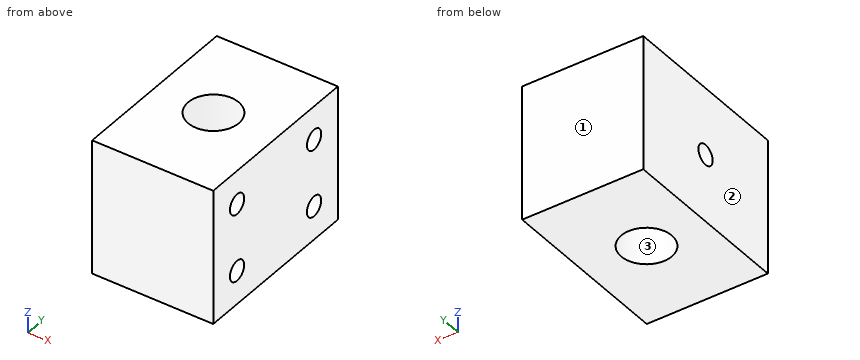
```python
from build123d import *

# Parameters (mm, degrees)
SKETCH1_W                            = 22.7965
SKETCH1_H                            = 33.263796714
SKETCH1_R                            = 4.7625
BOSS_EXTRUDE1_DEPTH                  = 25.4
SET_SCREW_10_24_TAPPED_HOLE1_REACH   = 49.658
SET_SCREW_10_24_TAPPED_HOLE1_BORE_R  = 1.89865
MOUNT_SCREW_10_24_TAPPED_HOLE2_D     = 3.7973
MOUNT_SCREW_10_24_TAPPED_HOLE2_DEPTH = 12.954
MOUNT_SCREW_10_24_TAPPED_HOLE2_TIP   = 1.140824014


with BuildPart() as part:
    # Sketch1 → Boss-Extrude1 (new body)
    with BuildSketch(Plane.XY):
        with Locations((11.39825, 16.631898357)):
            Rectangle(SKETCH1_W, SKETCH1_H)
        with Locations((11.1125, 16.631898357)):
            Circle(SKETCH1_R, mode=Mode.SUBTRACT)
    extrude(amount=BOSS_EXTRUDE1_DEPTH)

    # set screw #10-24 Tapped Hole1 bore → set screw #10-24 Tapped Hole1 (cut, up to next)
    with BuildSketch(Plane.ZY, mode=Mode.PRIVATE) as set_screw_10_24_tapped_hole1_sk1:
        with Locations((12.7, 16.631898357)):
            Circle(SET_SCREW_10_24_TAPPED_HOLE1_BORE_R)
    set_screw_10_24_tapped_hole1_tool1 = extrude(set_screw_10_24_tapped_hole1_sk1.sketch, amount=-SET_SCREW_10_24_TAPPED_HOLE1_REACH, mode=Mode.PRIVATE) & part.part
    add(set_screw_10_24_tapped_hole1_tool1.solids().sort_by_distance((0, 16.631898, 12.7))[0], mode=Mode.SUBTRACT)

    # mount screw #10-24 Tapped Hole2
    with Locations(Plane(origin=(22.7965, 0, 0), x_dir=(0, 0, -1), z_dir=(1, 0, 0))):
        with Locations((-19.05, 26.913796714), (-6.35, 26.913796714), (-19.05, 6.35), (-6.35, 6.35)):
            Hole(MOUNT_SCREW_10_24_TAPPED_HOLE2_D / 2, depth=MOUNT_SCREW_10_24_TAPPED_HOLE2_DEPTH)
            with Locations((0, 0, -(MOUNT_SCREW_10_24_TAPPED_HOLE2_DEPTH + MOUNT_SCREW_10_24_TAPPED_HOLE2_TIP / 2))):  # 118° drill point
                Cone(0, MOUNT_SCREW_10_24_TAPPED_HOLE2_D / 2, MOUNT_SCREW_10_24_TAPPED_HOLE2_TIP, mode=Mode.SUBTRACT)


solid = part.part
```
Design review of the part built by this model. Coordinates are the model's own, in mm. Face numbers are marked on the shaded views. Give positions to 0.01 mm unless a question says otherwise; leave off trailing zeros. Order: outer loops, then holes, each group sorted by start corner. A loop starts at its lowest first (then second) coordinate and runs counter-clockwise, first axis right, second up. Notation, with made-up numbers: M 5.5,-5 L 27.5,-5 A10 cw 27.5,4 Z; hole C 6,57 d2. An arc over 180 degrees is marked long. One line per question, with ' | ' between items. Start each with the question number.
Q1. We need section B-B (y = 19). Write out the cut boundary in (x, z).
Q2. For pin 1 Ø3.5 at (y, z) = (26.91, 19.05) entering from +X; pin 2 Ø6 at (y, z) = (23.5, 17.5) entering from -X; pin 3 Ø5.5 at (x, y) = (11.11, 16.63) entering from +Z; pin 4 Ø2.5 at (y, z) = (16.63, 12.7) entering from -X, all flat-tipped, find the tip position at first contact; note any pin that passes through.
Q3. The part is to be moulded in two halves that separate along Y. For the marked faces 1, 2 and 3, say which applies: +Y half, -Y half, draft (parallel to the pull), parting line (faces both ways), or undercut.
Q4. We need section A-A (x = 10.75). Write out the cut boundary in (y, z), plus the area to 3 significant figures.
Q5. We need section D-D (x = 19.25). Write out the cut boundary in (y, z).
Q6. We need section C-C (z = 12.7). Write out the cut boundary in (x, y) (1 decimal).
Q7. For L1, parallel to Z at x = 13.75, y = 6.35; L2, parallel to Y at x = 3.75, z = 12.7; L3, parallel to Z at x = 13.5, y = 28, list the stretches that pass through material, from the lowest coordinate up. Write a range as [from, to].
Returned:
1) outline: M 0,0 L 6.98,0 L 6.98,25.4 L 0,25.4 Z; M 15.24,0 L 22.8,0 L 22.8,25.4 L 15.24,25.4 Z
2) pin 1: x = 9.76 | pin 2: x = 0 | pin 3: through | pin 4: x = 15.71
3) face 1: +Y half | face 2: draft | face 3: undercut
4) outline: M 0,0 L 11.88,0 L 11.88,25.4 L 0,25.4 Z; M 21.38,0 L 33.26,0 L 33.26,25.4 L 21.38,25.4 Z; hole C 6.35,6.35 d3.8; hole C 6.35,19.05 d3.8; hole C 26.91,6.35 d3.8; hole C 26.91,19.05 d3.8 | area: 558 mm2
5) outline: M 0,0 L 33.26,0 L 33.26,25.4 L 0,25.4 Z; hole C 6.35,6.35 d3.8; hole C 6.35,19.05 d3.8; hole C 26.91,6.35 d3.8; hole C 26.91,19.05 d3.8
6) outline: M 0,0 L 22.8,0 L 22.8,33.3 L 0,33.3 L 0,18.5 L 6.7,18.5 A4.8 cw long 6.7,14.7 L 0,14.7 Z
7) L1: [0, 4.45], [8.25, 17.15], [20.95, 25.4] | L2: [0, 14.73], [18.53, 33.26] | L3: [0, 4.79], [7.91, 17.49], [20.61, 25.4]
